Build history of the part. All positions in model axes, mm. Coordinates: 2 decimals unless noted, no trailing zeros. Loops run counter-clockwise (first coordinate to the right, second up) from the corner with the lowest first, then second, coordinate; pieces in that order, holes last. Notation, with made-up numbers: M -33,-15 L -7,-15 A22 ccw -7,19 Z; hole C -1.75,14.25 d5. An arc over 180 degrees is marked long. Write each question's results on one line, items separated by ' | '. Start each with the question number.
from build123d import *

# Parameters (mm, degrees)
CROQUIS1_R              = 1.5
CROQUIS1_R_2            = 4
SALIENTE_EXTRUIR1_DEPTH = 2


with BuildPart() as part:
    # Croquis1 → Saliente-Extruir1 (new body)
    with BuildSketch(Plane.XY):
        with BuildLine():
            Line((23.828427125, -18.671572875), (20.328427125, -22.171572875))
            ThreePointArc((20.328427125, -22.171572875), (17.5, -23.343145751), (14.671572875, -22.171572875))
            Line((14.671572875, -22.171572875), (-6.328427125, -1.171572875))
            ThreePointArc((-6.328427125, -1.171572875), (-7.19551813, 0.12612052), (-7.5, 1.656854249))
            Line((-7.5, 1.656854249), (-7.5, 21))
            ThreePointArc((-7.5, 21), (-6.328427125, 23.828427125), (-3.5, 25))
            Line((-3.5, 25), (21, 25))
            ThreePointArc((21, 25), (23.828427125, 23.828427125), (25, 21))
            Line((25, 21), (25, -15.843145751))
            ThreePointArc((25, -15.843145751), (24.69551813, -17.37387948), (23.828427125, -18.671572875))
        make_face()
        Circle(CROQUIS1_R, mode=Mode.SUBTRACT)
        with Locations((17.5, -17.5)):
            Circle(CROQUIS1_R, mode=Mode.SUBTRACT)
        with Locations((0.625, 16.25)):
            Circle(CROQUIS1_R_2, mode=Mode.SUBTRACT)
        with Locations((16.875, 16.25)):
            Circle(CROQUIS1_R_2, mode=Mode.SUBTRACT)
    extrude(amount=SALIENTE_EXTRUIR1_DEPTH)


solid = part.part
1. Band-saw the part on A-A, the plane y = 16.25. List the corners of the cut face in (x, z) (3 decimals).
2. Pin check, flat tip, straight feed: pin 1 (2.5 mm diameter, centred on x = 17.5, y = -17.5, fed in from -Z). Stop position of the tip, or through.
3. Band-saw the part on C-C, the plane z = 1.1. List the corners of the cut face in (x, y) (3 decimals), plus the area to 3 significant figures.
4. Wall check: line 1 along X through (y, z) = (18, 1.55); line 2 along X through (y, z) = (19, 0.1); line 3 along Y through (x, z) = (-2, 1.1). Give the ranges that are in metal, low to high.
5. Band-saw the part on D-D, the plane y = -17.5. List the corners of the cut face in (x, z).
6. Mould opens along Y. For faces 1 (the cylindrical face through (13.927, 18.953, 0.986)), 2 (the flat face through (22.1, -20.4, 1)), 3 (the flat face through (9, 25, 1)), 4 (the flat face through (9, 7, 0)) say: +Y half, -Y half, draft (parallel to the pull), parting line (faces both ways), or undercut.
7. Band-saw the part on B-B, the plane x = 0. List the corners of the cut face in (y, z), plus the area to 3 significant figures.
Checked values:
1) outline: M -7.5,0 L -3.375,0 L -3.375,2 L -7.5,2 Z; M 4.625,0 L 12.875,0 L 12.875,2 L 4.625,2 Z; M 20.875,0 L 25,0 L 25,2 L 20.875,2 Z
2) pin 1: through
3) outline: M -7.5,1.657 A4 ccw -6.328,-1.172 L 14.672,-22.172 A4 ccw 20.328,-22.172 L 23.828,-18.672 A4 ccw 25,-15.843 L 25,21 A4 ccw 21,25 L -3.5,25 A4 ccw -7.5,21 Z; hole C 0.625,16.25 d8; hole C 0,0 d3; hole C 16.875,16.25 d8; hole C 17.5,-17.5 d3 | area: 1,160 mm²
4) line 1: -7.5 to -2.97, 4.22 to 13.28, 20.47 to 25 | line 2: -7.5 to -2.28, 3.53 to 13.97, 19.78 to 25 | line 3: -5.5 to 13.23, 19.27 to 25
5) outline: M 10,0 L 16,0 L 16,2 L 10,2 Z; M 19,0 L 24.64,0 L 24.64,2 L 19,2 Z
6) face 1: undercut | face 2: -Y half | face 3: +Y half | face 4: draft
7) outline: M -7.5,0 L -1.5,0 L -1.5,2 L -7.5,2 Z; M 1.5,0 L 12.3,0 L 12.3,2 L 1.5,2 Z; M 20.2,0 L 25,0 L 25,2 L 20.2,2 Z | area: 43.2 mm²
